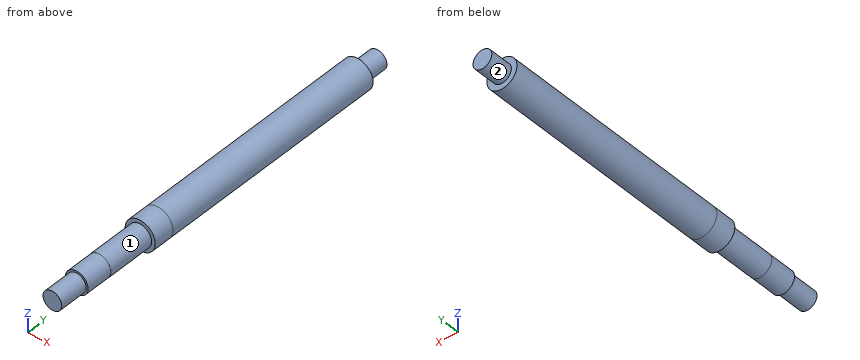
Autodesk Inventor part; units mm, degrees
ref_plane "YZ Plane" through (0, 0, 0) normal (1, 0, 0) x (0, 1, 0)
ref_plane "XZ Plane" through (0, 0, 0) normal (0, 1, 0) x (-1, 0, 0)
ref_plane "XY Plane" through (0, 0, 0) normal (0, 0, 1) x (1, 0, 0)
sketch "Sketch1" plane through (0, 0, 0) normal (0, 1, 0) x (-1, 0, 0)
  circle A0 centre (0, 0) radius 8
  dimension "d0" = 16
extrude "Extrusion1" add sketch "Sketch1" along normal blind 200
sketch "Sketch2" plane through (0, 0, 0) normal (0, -1, 0) x (1, 0, 0)
  circle A0 centre (0, 0) radius 8
extrude "Extrusion2" cut sketch "Sketch2" against normal blind 50
sketch "Sketch3" plane through (0, 50, 0) normal (0, -1, 0) x (1, 0, 0)
  circle A0 centre (0, 0) radius 8
extrude "Extrusion3" add sketch "Sketch3" along normal blind 50
sketch "Sketch4" plane through (0, 0, 0) normal (0, -1, 0) x (1, 0, 0)
  circle A0 centre (0, 0) radius 8
  circle A1 centre (0, 0) radius 6
  dimension "d7" = 12
extrude "Extrusion4" cut sketch "Sketch4" against normal blind 14
thread "Thread1"
sketch "Sketch6" plane through (0, 14, 0) normal (0, -1, 0) x (1, 0, 0)
  circle A0 centre (0, 0) radius 8
  circle A1 centre (0, 0) radius 6.05
  dimension "d13" = 12.1
extrude "Extrusion5" cut sketch "Sketch6" against normal blind 25
sketch "Sketch7" plane through (0, 0, 0) normal (0, -1, 0) x (1, 0, 0)
  circle A0 centre (0, 0) radius 6
  circle A1 centre (0, 0) radius 5
  dimension "d16" = 10
extrude "Extrusion6" add sketch "Sketch7" along normal blind 15 contours A1
sketch "Sketch8" plane through (0, 200, 0) normal (0, 1, 0) x (1, 0, 0)
  circle A0 centre (0, 0) radius 8
extrude "Extrusion7" cut sketch "Sketch8" against normal blind 27.101
sketch "Sketch9" plane through (0, 172.899, 0) normal (0, 1, 0) x (1, 0, 0)
  circle A0 centre (0, 0) radius 8
  circle A1 centre (0, 0) radius 5
  dimension "d21" = 10
extrude "Extrusion8" add sketch "Sketch9" along normal blind 12 contours A1
properties part number "1605_200mm"
Can you work these out from the model? Positions are in its coordinate system, mm. Face numbers are marked on the shaded views. A direction names the side the tool comes from. Round coordinates to 2 decimals unless told otherwise and drop trailing zeros. Loops run counter-clockwise (first coordinate to the right, second up) from the corner with the lowest first, then second, coordinate; pieces in that order, holes last. Notation, with made-up numbers: (20.25, 45) -> (55.25, 45) arc R18 ccw to (55.25, 70) -> close; hole circle Ø11 at (-16, 53). An arc over 180 degrees is marked (long way). One line per item, written item: value. Start each with the question number.
1. For pin 1 (1.5 mm diameter, centred on x = -4.5, y = 136, fed in from -Z); pin 2 (1.5 mm diameter, centred on y = 96, z = 4.5, fed in from -X); pin 3 (3 mm diameter, centred on y = 50.5, z = -2, fed in from +X), each with a flat end and sliding along its axis, tell me the tip position at first contact or that it passes through.
2. If I drill on probe 1 along Y at (x, z) = (6.75, -1); probe 2 along X at (y, z) = (67.5, 5.25); probe 3 along Z at (x, y) = (6.25, 77.5), over which ranges is the centre line in solid material (lowest first)?
3. If we section it at B-B, the plane z = 1.75: Write out the boundary of the cut face in (x, y).
4. If we section it at A-A, the plane x = 0: Write out the boundary of the cut face in (y, z).
5. If we section it at C-C, the plane y = 75: Write out the boundary of the cut face in (x, z), then the cut area to 3 significant figures.
6. For the marked faces 1 and 2, which set-ups out of +Z, -Z, +X, -X, +Y, -Y let a thin tool reach every point of the face, with its end or its side?
Calculated:
1. pin 1: stops at z = -7.07
1. pin 2: stops at x = -7.07
1. pin 3: stops at x = 7.98
2. probe 1: y = 39 to 172.9
2. probe 2: x = -6.04 to 6.04
2. probe 3: z = -4.99 to 4.99
3. outline: (-7.81, 39) -> (-5.79, 39) -> (-5.79, 14) -> (-5.74, 14) -> (-5.74, 0) -> (-4.68, 0) -> (-4.68, -15) -> (4.68, -15) -> (4.68, 0) -> (5.74, 0) -> (5.74, 14) -> (5.79, 14) -> (5.79, 39) -> (7.81, 39) -> (7.81, 172.9) -> (4.68, 172.9) -> (4.68, 184.9) -> (-4.68, 184.9) -> (-4.68, 172.9) -> (-7.81, 172.9) -> close
4. outline: (-15, -5) -> (0, -5) -> (0, -6) -> (14, -6) -> (14, -6.05) -> (39, -6.05) -> (39, -8) -> (172.9, -8) -> (172.9, -5) -> (184.9, -5) -> (184.9, 5) -> (172.9, 5) -> (172.9, 8) -> (39, 8) -> (39, 6.05) -> (14, 6.05) -> (14, 6) -> (0, 6) -> (0, 5) -> (-15, 5) -> close
5. outline: circle Ø16 at (0, 0)
5. area: 201 mm²
6. face 1: -Y
6. face 2: +Y
